Could you check a few things on this model? Use its own coordinates, in mm. A direction names the side the tool comes from. Round coordinates to 2 decimals unless told otherwise and drop trailing zeros. Write each loop counter-clockwise with the first axis right and the second up, starting at its lowest first coordinate (ties: lowest second). Pieces come first, ordered by that corner, then holes. Notation, with made-up numbers: M 18.5,84 L 62.5,84 A21 cw 62.5,89 Z; hole C -23.5,39.25 d11. An arc over 180 degrees is marked long. One line per item, written item: value. Start each with the question number.
(1) If I drill on L1, parallel to Y at x = 19.5, z = 16; L2, parallel to Z at x = 52, y = 1.5; L3, parallel to Z at x = 80, y = 133.5, over which ranges is the centre line in solid material (lowest first)?
(2) I want a section at C-C on y = 18. Please give me the cut outline in (x, z).
(3) I want a section at A-A on z = 23.5. Please give me the cut outline in (x, y), and give its area (3 significant figures).
(4) I'm going to push flat-ended pins straight in: pin 1 Ø1.5 at (x, z) = (51.9, 5.3) entering from +Y; pin 2 Ø4 at (x, y) = (-0.7, 183.4) entering from -Z; pin 3 Ø10.5 at (x, y) = (-11, 184) entering from +Z. Where does each tip first touch, or does it pass through?
(5) Which directions (+Z, -Z, +X, -X, +Y, -Y) give clear straight access to the entire face, cutting with the end or side of a thin tool? Please do faces 1 (the face through (81.3, 86, 16)), 2 (the face through (1, 175.403, 5)), 3 (the face through (68.25, 180.21, 16.31)), 4 (the face through (49.9, 1.6, 19.5)).
(6) Thinking about a two-plate mould opening in Y: for faces 5 (the face through (84.3, 72, 16)), 6 (the face through (40, -25, 16)), 7 (the face through (43, -28, 16)), which applies, released by +Y, released by -Y, zero draft, split by the parting line, or undercut?
(7) I want a section at B-B on y = 136.5. Please give me the cut outline in (x, z), and give its area (3 significant figures).
```python
from build123d import *

# Parameters (mm, degrees)
EXTRUDE_6_DEPTH      = 33
CUT_EXTRUDE_START    = 3
CUT_EXTRUDE_2_DEPTH  = 27
EXTRUDE_START        = 6.5
SKETCH_7_W           = 26
SKETCH_7_H           = 13
EXTRUDE_7_DEPTH      = 20
EXTRUDE_START_2      = 1.5
SKETCH_11_W          = 13
SKETCH_11_H          = 2.5
EXTRUDE_15_DEPTH     = 30
CUT_EXTRUDE_START_2  = 180
SKETCH_12_R          = 1
CUT_EXTRUDE_3_DEPTH  = 10
SKETCH_13_R          = 1.5
CUT_EXTRUDE_4_DEPTH  = 30
SKETCH_14_W          = 7
SKETCH_14_H          = 2
CUT_EXTRUDE_5_DEPTH  = 30
EXTRUDE_START_3      = 11.5
SKETCH_15_W          = 67.299618531
SKETCH_15_H          = 10
EXTRUDE_16_DEPTH     = 10
SKETCH_16_W          = 8.5
SKETCH_16_H          = 10
CUT_EXTRUDE_6_DEPTH  = 79
CUT_EXTRUDE_START_3  = 16.5
SKETCH_17_R          = 3
CUT_EXTRUDE_7_DEPTH  = 75
CUT_EXTRUDE_START_4  = 13
SKETCH_18_R          = 1.5
CUT_EXTRUDE_9_DEPTH  = 5
SKETCH_20_R          = 1.25
SKETCH_20_W          = 16.6
SKETCH_20_H          = 24.7
CUT_EXTRUDE_10_DEPTH = 5
SKETCH_21_R          = 5
CUT_EXTRUDE_11_DEPTH = 5


with BuildPart() as part:
    # Эскиз1 → Бобышка-Вытянуть6 (new body)
    with BuildSketch(Plane.XY):
        with BuildLine():
            Line((4.299618531, 175.402841826), (4.299618531, 188.402841826))
            Line((4.299618531, 188.402841826), (64.299618531, 188.402841826))
            Line((64.299618531, 188.402841826), (84.299618531, 168.402841826))
            Line((84.299618531, 168.402841826), (84.299618531, 0))
            Line((84.299618531, 0), (84.299618531, -28))
            Line((84.299618531, -28), (0, -28))
            Line((0, -28), (0, 0))
            ThreePointArc((0, 0), (37.229295141, 21.561020186), (55.173142182, 60.662380285))
            ThreePointArc((55.173142182, 60.662380285), (56.797307883, 87.162380285), (55.173142182, 113.662380285))
            ThreePointArc((55.173142182, 113.662380285), (38.726552267, 151.940422917), (4.299618531, 175.402841826))
        make_face()
    extrude(amount=EXTRUDE_6_DEPTH)

    # Эскиз5 → Вырез-Вытянуть2 (cut)
    with BuildSketch(Plane.XY.offset(CUT_EXTRUDE_START)):
        Polygon((-18.700381469, -25), (81.299618531, -25), (81.299618531, -3.5), (14, -3.5), (14, 6.5), (81.299618531, 6.5), (81.299618531, 167.160201139), (63.056977844, 185.402841826), (23.056977844, 185.402841826), (23.056977844, 175.402841826), (4.299618531, 175.402841826), (6.299618531, 167.160201139), (-18.700381469, 167.160201139), align=None)
    extrude(amount=CUT_EXTRUDE_2_DEPTH, mode=Mode.SUBTRACT)

    # Эскиз7 → Бобышка-Вытянуть7 (add)
    with BuildSketch(Plane.XY.offset(EXTRUDE_START)):
        with Locations((-8.700381469, 181.902841826)):
            Rectangle(SKETCH_7_W, SKETCH_7_H)
    extrude(amount=EXTRUDE_7_DEPTH)

    # Эскиз11 → Бобышка-Вытянуть15 (add)
    with BuildSketch(Plane.XY.offset(EXTRUDE_START_2)):
        with Locations((3.799618531, 174.152841826)):
            Rectangle(SKETCH_11_W, SKETCH_11_H)
    extrude(amount=EXTRUDE_15_DEPTH)

    # Эскиз12 → Вырез-Вытянуть3 (cut)
    with BuildSketch(Plane(origin=(0, 0, 0), x_dir=(1, 0, 0), z_dir=(0, 1, 0)).offset(CUT_EXTRUDE_START_2)):
        with Locations((1.142696527, -3.5)):
            Circle(SKETCH_12_R)
        with Locations((1.142696527, -29.5)):
            Circle(SKETCH_12_R)
    extrude(amount=-CUT_EXTRUDE_3_DEPTH, mode=Mode.SUBTRACT)

    # Эскиз13 → Вырез-Вытянуть4 (cut)
    with BuildSketch(Plane.XY):
        with Locations((-0.700381469, 183.402841826)):
            Circle(SKETCH_13_R)
    extrude(amount=CUT_EXTRUDE_4_DEPTH, mode=Mode.SUBTRACT)

    # Эскиз14 → Вырез-Вытянуть5 (cut)
    with BuildSketch(Plane.XY):
        with Locations((-18.200381469, 187.402841826)):
            Rectangle(SKETCH_14_W, SKETCH_14_H)
    extrude(amount=CUT_EXTRUDE_5_DEPTH, mode=Mode.SUBTRACT)

    # Эскиз15 → Бобышка-Вытянуть16 (add)
    with BuildSketch(Plane.XY.offset(EXTRUDE_START_3)):
        with Locations((47.649809266, 1.5)):
            Rectangle(SKETCH_15_W, SKETCH_15_H)
    extrude(amount=EXTRUDE_16_DEPTH)

    # Эскиз16 → Вырез-Вытянуть6 (cut)
    with BuildSketch(Plane(origin=(0, 0, 0), x_dir=(0, 0, -1), z_dir=(1, 0, 0))):
        with Locations((-7.25, 1.5)):
            Rectangle(SKETCH_16_W, SKETCH_16_H)
        with Locations((-25.75, 1.5)):
            Rectangle(SKETCH_16_W, SKETCH_16_H)
    extrude(amount=CUT_EXTRUDE_6_DEPTH, mode=Mode.SUBTRACT)

    # Эскиз17 → Вырез-Вытянуть7 (cut)
    with BuildSketch(Plane(origin=(0, 0, 0), x_dir=(0, 0, -1), z_dir=(1, 0, 0)).offset(CUT_EXTRUDE_START_3)):
        with Locations((-16.5, 1.5)):
            Circle(SKETCH_17_R)
    extrude(amount=CUT_EXTRUDE_7_DEPTH, mode=Mode.SUBTRACT)

    # Эскиз18 → Вырез-Вытянуть9 (cut)
    with BuildSketch(Plane(origin=(0, 0, 0), x_dir=(0, 0, -1), z_dir=(1, 0, 0)).offset(CUT_EXTRUDE_START_4)):
        with Locations((-16.5, 1.5)):
            Circle(SKETCH_18_R)
    extrude(amount=CUT_EXTRUDE_9_DEPTH, mode=Mode.SUBTRACT)

    # Эскиз20 → Вырез-Вытянуть10 (cut)
    with BuildSketch(Plane(origin=(0, 188.402841826, 0), x_dir=(1, 0, 0), z_dir=(0, 1, 0))):
        with Locations((51.9, -5.3)):
            Circle(SKETCH_20_R)
        with Locations((51.9, -27.7)):
            Circle(SKETCH_20_R)
        with Locations((30, -5.3)):
            Circle(SKETCH_20_R)
        with Locations((30, -27.7)):
            Circle(SKETCH_20_R)
        with Locations((40.95, -16.5)):
            Rectangle(SKETCH_20_W, SKETCH_20_H)
    extrude(amount=-CUT_EXTRUDE_10_DEPTH, mode=Mode.SUBTRACT)

    # Эскиз21 → Вырез-Вытянуть11 (cut)
    with BuildSketch(Plane(origin=(126.351230179, 126.351230179, 0), x_dir=(0, 0, -1), z_dir=(0.707106781, 0.707106781, 0))):
        with Locations((-16.5, 73.612095136)):
            Circle(SKETCH_21_R)
    extrude(amount=-CUT_EXTRUDE_11_DEPTH, mode=Mode.SUBTRACT)


solid = part.part
```
Found:
1. L1: y = -28 to -25, -3.5 to -1.46, 4.46 to 6.5, 175.4 to 188.4
1. L2: z = 0 to 3, 11.5 to 13.5, 19.5 to 21.5, 30 to 33
1. L3: z = 0 to 3, 30 to 33
2. outline: M 33.75,0 L 84.3,0 L 84.3,33 L 33.75,33 L 33.75,30 L 81.3,30 L 81.3,3 L 33.75,3 Z
3. outline: M -21.7,175.4 L -2.7,175.4 L -2.7,172.9 L 10.3,172.9 L 10.3,175.4 L 23.06,175.4 L 23.06,185.4 L 32.65,185.4 L 32.65,188.4 L -14.7,188.4 L -14.7,186.4 L -21.7,186.4 Z; M 0,-28 L 84.3,-28 L 84.3,168.4 L 64.3,188.4 L 49.25,188.4 L 49.25,185.4 L 63.06,185.4 L 81.3,167.16 L 81.3,6.5 L 79,6.5 L 79,-3.5 L 81.3,-3.5 L 81.3,-25 L 0,-25 Z; hole C -0.7,183.4 d3
3. area: 1,600 mm²
4. pin 1: stops at y = -25
4. pin 2: stops at z = 6.5
4. pin 3: stops at z = 26.5
5. face 1: -X
5. face 2: -Z, -X, +Y
5. face 3: none
5. face 4: +X
6. face 5: zero draft
6. face 6: undercut
6. face 7: released by -Y
7. outline: M 48.54,0 L 84.3,0 L 84.3,33 L 48.54,33 L 48.54,30 L 81.3,30 L 81.3,3 L 48.54,3 Z
7. area: 296 mm²
